```python
from build123d import *

# Parameters (mm, degrees)
F0_W     = 165
F0_H     = 100
F1_DEPTH = 2.5
F2_R     = 5.5
F2_W     = 10
F2_H     = 30
F2_R_2   = 2
F3_DEPTH = 25


with BuildPart() as f1:
    # F0 (on Top) → F1 (new body)
    with BuildSketch(Plane.XY):
        Rectangle(F0_W, F0_H)
    extrude(amount=F1_DEPTH)

    # F2 (on face) → F3 (cut)
    with BuildSketch(Plane.XY.offset(2.5)):
        with Locations((-8, 14.5)):
            Circle(F2_R)
        with Locations((-8, -0.5)):
            Circle(F2_R)
        with Locations((19.125108, -15.5)):
            Circle(F2_R)
        with Locations((-38.5, 15)):
            Rectangle(F2_W, F2_H)
        with Locations((-70.5, 14.5)):
            Circle(F2_R_2)
        with Locations((-70.5, -0.5)):
            Circle(F2_R_2)
    extrude(amount=-F3_DEPTH, mode=Mode.SUBTRACT)


solid = f1.part
```
CAD build for the part. Positions are in the model's coordinates, mm. Coordinates: 2 decimals unless noted, no trailing zeros. Loops run counter-clockwise (first coordinate to the right, second up) from the corner with the lowest first, then second, coordinate; pieces in that order, holes last. Notation, with made-up numbers: (-36.75, -13.5) - (-2.75, -13.5) arc R23 cw to (-2.75, 6.5) - close; hole circle Ø7 at (-7, -24). An arc over 180 degrees is marked (long way). Return JSON: item names as keys, results as strings.
1. Band-saw the part on C-C (y = -15.5). Give the cut face in (x, z), and give its area (3 significant figures).
Result:
{"outline": "(-82.5, 0) - (13.63, 0) - (13.63, 2.5) - (-82.5, 2.5) - close; (24.63, 0) - (82.5, 0) - (82.5, 2.5) - (24.63, 2.5) - close", "area": "385 mm2"}
2. Probe L1, parallel to Y at x = -8, z = 0.6; L2, parallel to X at y = 27.5, z = 0.75; L3, parallel to X at y = -12, z = 2. List the from-to ranges inside material, lowest first. Write a range as from..to.
Result:
{"L1": "y = -50..-6, 5..9, 20..50", "L2": "x = -82.5..-43.5, -33.5..82.5", "L3": "x = -82.5..14.88, 23.37..82.5"}
3. Drop a flat-ended pin along its axis: pin 1 (6.5 mm diameter, centred on x = -8, y = 14.5, fed in from +Z). Give the stop position or say it passes through.
Result:
{"pin 1": "passes through"}
4. Mould opens along Y. For faces 1 (the flat face through (-1, 1, 0)), 2 (the cylindrical face through (-68.592, 0.101, 1.268)) say: released by +Y, released by -Y, zero draft, split by the parting line, or undercut.
Result:
{"face 1": "zero draft", "face 2": "undercut"}
5. Band-saw the part on A-A (x = -8). Give the cut face in (y, z), and give its area (3 significant figures).
Result:
{"outline": "(-50, 0) - (-6, 0) - (-6, 2.5) - (-50, 2.5) - close; (5, 0) - (9, 0) - (9, 2.5) - (5, 2.5) - close; (20, 0) - (50, 0) - (50, 2.5) - (20, 2.5) - close", "area": "195 mm2"}
6. Band-saw the part on D-D (z = 0.85). Give the cut face in (x, y), and give its area (3 significant figures).
Result:
{"outline": "(-82.5, -50) - (82.5, -50) - (82.5, 50) - (-82.5, 50) - close; hole circle Ø4 at (-70.5, -0.5); hole circle Ø4 at (-70.5, 14.5); hole (-43.5, 0) - (-33.5, 0) - (-33.5, 30) - (-43.5, 30) - close; hole circle Ø11 at (-8, -0.5); hole circle Ø11 at (-8, 14.5); hole circle Ø11 at (19.13, -15.5)", "area": "15,900 mm2"}
7. Band-saw the part on B-B (y = 14.5). Give the cut face in (x, z), and give its area (3 significant figures).
Result:
{"outline": "(-82.5, 0) - (-72.5, 0) - (-72.5, 2.5) - (-82.5, 2.5) - close; (-68.5, 0) - (-43.5, 0) - (-43.5, 2.5) - (-68.5, 2.5) - close; (-33.5, 0) - (-13.5, 0) - (-13.5, 2.5) - (-33.5, 2.5) - close; (-2.5, 0) - (82.5, 0) - (82.5, 2.5) - (-2.5, 2.5) - close", "area": "350 mm2"}
